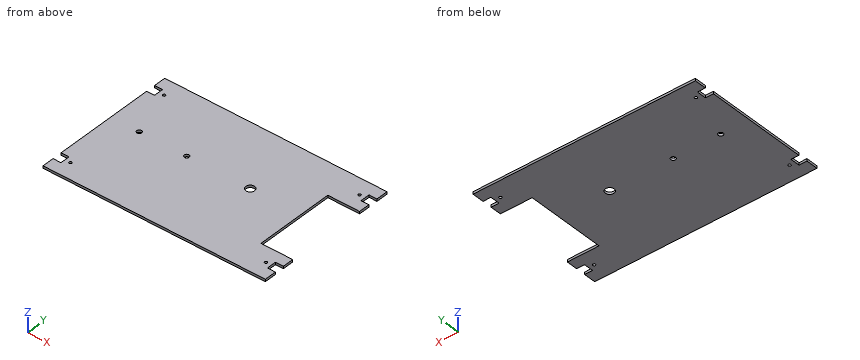
from build123d import *

# Parameters (mm, degrees)
BOSS_EXTRUDE1_DEPTH = 1.5
SKETCH2_R           = 1.5
SKETCH2_R_2         = 2.75
CUT_EXTRUDE1_DEPTH  = 1.5
SKETCH5_W           = 5
SKETCH5_H           = 6
SKETCH5_R           = 0.85
CUT_EXTRUDE5_DEPTH  = 167.982783544


with BuildPart() as part:
    # Sketch1 → Boss-Extrude1 (new body)
    with BuildSketch(Plane.XY):
        Polygon((140, 0), (0, 0), (0, -91), (140, -91), (140, -70.5), (120, -70.5), (120, -20.5), (140, -20.5), align=None)
    extrude(amount=BOSS_EXTRUDE1_DEPTH)

    # Sketch2 → Cut-Extrude1 (cut)
    with BuildSketch(Plane.XY.offset(1.5)):
        with Locations((18, -40.4)):
            Circle(SKETCH2_R)
        with Locations((48, -40.5)):
            Circle(SKETCH2_R)
        with Locations((88, -40.5)):
            Circle(SKETCH2_R_2)
    extrude(amount=-CUT_EXTRUDE1_DEPTH, mode=Mode.SUBTRACT)

    # Sketch5 → Cut-Extrude5 (cut, through all)
    with BuildSketch(Plane.XY.offset(1.5)):
        with Locations((2.5, -10.5)):
            Rectangle(SKETCH5_W, SKETCH5_H)
        with Locations((2.5, -80.5)):
            Rectangle(SKETCH5_W, SKETCH5_H)
        with Locations((137.5, -80.5)):
            Rectangle(SKETCH5_W, SKETCH5_H)
        with Locations((137.5, -10.5)):
            Rectangle(SKETCH5_W, SKETCH5_H)
        with Locations((8.45, -10.5)):
            Circle(SKETCH5_R)
        with Locations((8.45, -80.5)):
            Circle(SKETCH5_R)
        with Locations((131.55, -80.5)):
            Circle(SKETCH5_R)
        with Locations((131.55, -10.5)):
            Circle(SKETCH5_R)
    extrude(amount=-CUT_EXTRUDE5_DEPTH, mode=Mode.SUBTRACT)


solid = part.part
Geometry check sheet. Reference: the model listing, model coordinates, mm. Round coordinates to 2 decimals unless told otherwise and drop trailing zeros. Write each loop counter-clockwise with the first axis right and the second up, starting at its lowest first coordinate (ties: lowest second). Pieces come first, ordered by that corner, then holes. Notation, with made-up numbers: (73, 48.25) - (94, 48.25) arc R22 ccw to (94, 78.25) - close; hole circle Ø11 at (89, -19). An arc over 180 degrees is marked (long way). One line per item, written item: value.
1. Cross-section at A-A on x = 88. Record the boundary of the cut face in (y, z).
The answers:
outline: (-91, 0) - (-43.25, 0) - (-43.25, 1.5) - (-91, 1.5) - close; (-37.75, 0) - (0, 0) - (0, 1.5) - (-37.75, 1.5) - close
2. Cross-section at C-C on x = 18. Record the boundary of the cut face in (y, z).
The answers:
outline: (-91, 0) - (-41.9, 0) - (-41.9, 1.5) - (-91, 1.5) - close; (-38.9, 0) - (0, 0) - (0, 1.5) - (-38.9, 1.5) - close
3. Scan lines: L1, parallel to Y at x = 131.55, z = 0.95; L2, parallel to Y at x = 125.5, z = 0.6; L3, parallel to Y at x = 48, z = 1.25. Record each from-to range of solid material in increasing order.
The answers:
L1: y = -91 to -81.35, -79.65 to -70.5, -20.5 to -11.35, -9.65 to 0
L2: y = -91 to -70.5, -20.5 to 0
L3: y = -91 to -42, -39 to 0
4. Depth check by flat-ended pin: pin 1 Ø2.5 at (x, y) = (18, -40.4) entering from -Z. Enter the tip coordinate at first touch or a pass-through.
The answers:
pin 1: passes through
5. Cross-section at B-B on z = 0.65. Give the number of separate pieces and of enclosed holes in the cut face, and give its area (3 significant figures).
The answers:
separate pieces: 1
enclosed holes: 7
area: 11,600 mm^2
